Could you check a few things on this model? Use its own coordinates, in mm. Face numbers are marked on the shaded views. A direction names the side the tool comes from. Give positions to 0.01 mm unless a question says otherwise; leave off trailing zeros. One line per question, with ' | ' between items.
from build123d import *

# Parameters (mm, degrees)
BOSS_EXTRUDE1_DEPTH     = 6.2
BOSS_EXTRUDE3_DEPTH     = 6.2
CUT_EXTRUDE5_DEPTH      = 59.510170056
CUT_EXTRUDE5_DEPTH_BACK = 59.510170056
SKETCH9_W               = 8.426821026
SKETCH9_H               = 53.817918331
CUT_EXTRUDE6_DEPTH      = 56.427921054
CUT_EXTRUDE6_DEPTH_BACK = 56.427921054
SKETCH10_W              = 41.255234225
SKETCH10_H              = 19.128366746


with BuildPart() as part:
    # Sketch1 → Boss-Extrude1 (new body)
    with BuildSketch(Plane.XY):
        with BuildLine():
            Line((-28, 0), (0, 0))
            Line((0, 0), (0, 10))
            Line((0, 10), (-7.1, 10))
            ThreePointArc((-7.1, 10), (-14.171067812, 12.928932188), (-17.1, 20))
            Line((-17.1, 20), (-17.1, 51))
            Line((-17.1, 51), (-20.1, 51))
            Line((-20.1, 51), (-20.1, 6))
            Line((-20.1, 6), (-24, 6))
            Line((-24, 6), (-24, 50))
            Line((-24, 50), (-28, 50))
            Line((-28, 50), (-28, 0))
        make_face()
    extrude(amount=BOSS_EXTRUDE1_DEPTH)

    # Sketch7 → Boss-Extrude3 (add)
    with BuildSketch(Plane.XY.offset(6.2)):
        with BuildLine():
            Line((-16.7, 50.6), (-15.7, 50.5))
            ThreePointArc((-15.7, 50.5), (-15.462165524, 50.365875857), (-15.4, 50.1))
            ThreePointArc((-15.4, 50.1), (-15.462165524, 49.834124143), (-15.7, 49.7))
            Line((-15.7, 49.7), (-16.7, 49.6))
            ThreePointArc((-16.7, 49.6), (-16.971392676, 49.471392676), (-17.1, 49.2))
            Line((-17.1, 49.2), (-17.1, 48.75))
            ThreePointArc((-17.1, 48.75), (-16.971392676, 48.478607324), (-16.7, 48.35))
            Line((-16.7, 48.35), (-15.7, 48.25))
            ThreePointArc((-15.7, 48.25), (-15.462165524, 48.115875857), (-15.4, 47.85))
            ThreePointArc((-15.4, 47.85), (-15.462165524, 47.584124143), (-15.7, 47.45))
            Line((-15.7, 47.45), (-16.7, 47.35))
            ThreePointArc((-16.7, 47.35), (-16.971392676, 47.221392676), (-17.1, 46.95))
            Line((-17.1, 46.95), (-17.1, 46.5))
            ThreePointArc((-17.1, 46.5), (-16.971392676, 46.228607324), (-16.7, 46.1))
            Line((-16.7, 46.1), (-15.7, 46))
            ThreePointArc((-15.7, 46), (-15.462165524, 45.865875857), (-15.4, 45.6))
            ThreePointArc((-15.4, 45.6), (-15.462165524, 45.334124143), (-15.7, 45.2))
            Line((-15.7, 45.2), (-16.7, 45.1))
            ThreePointArc((-16.7, 45.1), (-16.971392676, 44.971392676), (-17.1, 44.7))
            Line((-17.1, 44.7), (-17.1, 44.25))
            ThreePointArc((-17.1, 44.25), (-16.971392676, 43.978607324), (-16.7, 43.85))
            Line((-16.7, 43.85), (-15.7, 43.75))
            ThreePointArc((-15.7, 43.75), (-15.462165524, 43.615875857), (-15.4, 43.35))
            ThreePointArc((-15.4, 43.35), (-15.462165524, 43.084124143), (-15.7, 42.95))
            Line((-15.7, 42.95), (-16.7, 42.85))
            ThreePointArc((-16.7, 42.85), (-16.971392676, 42.721392676), (-17.1, 42.45))
            Line((-17.1, 42.45), (-17.1, 42))
            ThreePointArc((-17.1, 42), (-16.971392676, 41.728607324), (-16.7, 41.6))
            Line((-16.7, 41.6), (-15.7, 41.5))
            ThreePointArc((-15.7, 41.5), (-15.462165524, 41.365875857), (-15.4, 41.1))
            ThreePointArc((-15.4, 41.1), (-15.462165524, 40.834124143), (-15.7, 40.7))
            Line((-15.7, 40.7), (-16.7, 40.6))
            ThreePointArc((-16.7, 40.6), (-16.971392676, 40.471392676), (-17.1, 40.2))
            Line((-17.1, 40.2), (-17.1, 39.75))
            ThreePointArc((-17.1, 39.75), (-16.971392676, 39.478607324), (-16.7, 39.35))
            Line((-16.7, 39.35), (-15.7, 39.25))
            ThreePointArc((-15.7, 39.25), (-15.462165524, 39.115875857), (-15.4, 38.85))
            ThreePointArc((-15.4, 38.85), (-15.462165524, 38.584124143), (-15.7, 38.45))
            Line((-15.7, 38.45), (-16.7, 38.35))
            ThreePointArc((-16.7, 38.35), (-16.971392676, 38.221392676), (-17.1, 37.95))
            Line((-17.1, 37.95), (-17.1, 37.5))
            ThreePointArc((-17.1, 37.5), (-16.971392676, 37.228607324), (-16.7, 37.1))
            Line((-16.7, 37.1), (-15.7, 37))
            ThreePointArc((-15.7, 37), (-15.462165524, 36.865875857), (-15.4, 36.6))
            ThreePointArc((-15.4, 36.6), (-15.462165524, 36.334124143), (-15.7, 36.2))
            Line((-15.7, 36.2), (-16.7, 36.1))
            ThreePointArc((-16.7, 36.1), (-16.971392676, 35.971392676), (-17.1, 35.7))
            Line((-17.1, 35.7), (-17.1, 35.25))
            ThreePointArc((-17.1, 35.25), (-16.971392676, 34.978607324), (-16.7, 34.85))
            Line((-16.7, 34.85), (-15.7, 34.75))
            ThreePointArc((-15.7, 34.75), (-15.462165524, 34.615875857), (-15.4, 34.35))
            ThreePointArc((-15.4, 34.35), (-15.462165524, 34.084124143), (-15.7, 33.95))
            Line((-15.7, 33.95), (-16.7, 33.85))
            ThreePointArc((-16.7, 33.85), (-16.971392676, 33.721392676), (-17.1, 33.45))
            Line((-17.1, 33.45), (-17.1, 33))
            ThreePointArc((-17.1, 33), (-16.971392676, 32.728607324), (-16.7, 32.6))
            Line((-16.7, 32.6), (-15.7, 32.5))
            ThreePointArc((-15.7, 32.5), (-15.462165524, 32.365875857), (-15.4, 32.1))
            ThreePointArc((-15.4, 32.1), (-15.462165524, 31.834124143), (-15.7, 31.7))
            Line((-15.7, 31.7), (-16.7, 31.6))
            ThreePointArc((-16.7, 31.6), (-16.971392676, 31.471392676), (-17.1, 31.2))
            Line((-17.1, 31.2), (-17.1, 30.75))
            ThreePointArc((-17.1, 30.75), (-16.971392676, 30.478607324), (-16.7, 30.35))
            Line((-16.7, 30.35), (-15.7, 30.25))
            ThreePointArc((-15.7, 30.25), (-15.462165524, 30.115875857), (-15.4, 29.85))
            ThreePointArc((-15.4, 29.85), (-15.462165524, 29.584124143), (-15.7, 29.45))
            Line((-15.7, 29.45), (-16.7, 29.35))
            ThreePointArc((-16.7, 29.35), (-16.971392676, 29.221392676), (-17.1, 28.95))
            Line((-17.1, 28.95), (-17.1, 28.5))
            ThreePointArc((-17.1, 28.5), (-16.971392676, 28.228607324), (-16.7, 28.1))
            Line((-16.7, 28.1), (-15.7, 28))
            ThreePointArc((-15.7, 28), (-15.462165524, 27.865875857), (-15.4, 27.6))
            ThreePointArc((-15.4, 27.6), (-15.462165524, 27.334124143), (-15.7, 27.2))
            Line((-15.7, 27.2), (-16.7, 27.1))
            ThreePointArc((-16.7, 27.1), (-16.971392676, 26.971392676), (-17.1, 26.7))
            Line((-17.1, 26.7), (-17.1, 26.25))
            ThreePointArc((-17.1, 26.25), (-16.971392676, 25.978607324), (-16.7, 25.85))
            Line((-16.7, 25.85), (-15.7, 25.75))
            ThreePointArc((-15.7, 25.75), (-15.462165524, 25.615875857), (-15.4, 25.35))
            ThreePointArc((-15.4, 25.35), (-15.462165524, 25.084124143), (-15.7, 24.95))
            Line((-15.7, 24.95), (-16.7, 24.85))
            ThreePointArc((-16.7, 24.85), (-16.971392676, 24.721392676), (-17.1, 24.45))
            Line((-17.1, 24.45), (-17.1, 24))
            ThreePointArc((-17.1, 24), (-16.971392676, 23.728607324), (-16.7, 23.6))
            Line((-16.7, 23.6), (-15.7, 23.5))
            ThreePointArc((-15.7, 23.5), (-15.462165524, 23.365875857), (-15.4, 23.1))
            ThreePointArc((-15.4, 23.1), (-15.462165524, 22.834124143), (-15.7, 22.7))
            Line((-15.7, 22.7), (-16.7, 22.6))
            ThreePointArc((-16.7, 22.6), (-16.971392676, 22.471392676), (-17.1, 22.2))
            Line((-17.1, 22.2), (-17.1, 21.75))
            ThreePointArc((-17.1, 21.75), (-16.971392676, 21.478607324), (-16.7, 21.35))
            Line((-16.7, 21.35), (-15.7, 21.25))
            ThreePointArc((-15.7, 21.25), (-15.462165524, 21.115875857), (-15.4, 20.85))
            ThreePointArc((-15.4, 20.85), (-15.462165524, 20.584124143), (-15.7, 20.45))
            Line((-15.7, 20.45), (-16.7, 20.35))
            ThreePointArc((-16.7, 20.35), (-16.971392676, 20.221392676), (-17.1, 19.95))
            Line((-17.1, 19.95), (-17.956542174, 50.55))
            Line((-17.956542174, 50.55), (-17.1, 51))
            ThreePointArc((-17.1, 51), (-16.971392676, 50.728607324), (-16.7, 50.6))
        make_face()
    extrude(amount=-BOSS_EXTRUDE3_DEPTH)

    # Sketch9 → Cut-Extrude5 (cut, two sides: drawn at the far end of the back side and taken through both)
    with BuildSketch(Plane.XY.offset(6.2).offset(-CUT_EXTRUDE5_DEPTH_BACK)):
        with Locations((-25.017603177, 24.82792225)):
            Rectangle(SKETCH9_W, SKETCH9_H)
    extrude(amount=CUT_EXTRUDE5_DEPTH + CUT_EXTRUDE5_DEPTH_BACK, mode=Mode.SUBTRACT)

    # Sketch10 → Cut-Extrude6 (cut, two sides: drawn at the far end of the back side and taken through both)
    with BuildSketch(Plane.XY.offset(6.2).offset(-CUT_EXTRUDE6_DEPTH_BACK)):
        with Locations((-9.089657701, 8.103525919)):
            Rectangle(SKETCH10_W, SKETCH10_H)
    extrude(amount=CUT_EXTRUDE6_DEPTH + CUT_EXTRUDE6_DEPTH_BACK, mode=Mode.SUBTRACT)


solid = part.part
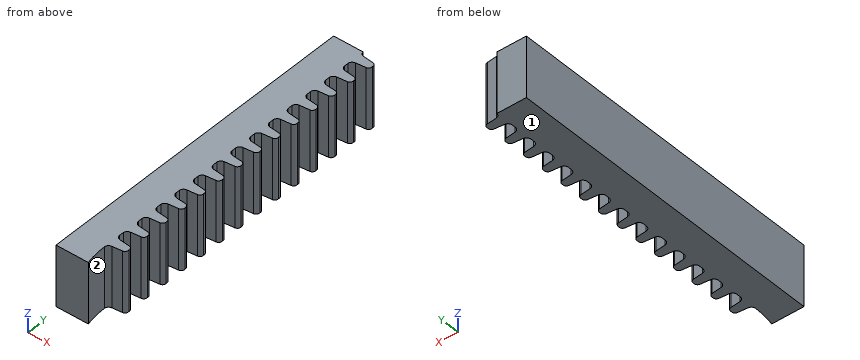
Q1. Will these pins go through, and if not, where does the flat tip stop? pin 1 (0.5 mm diameter, centred on y = 42, z = 3, fed in from +X); pin 2 (0.5 mm diameter, centred on y = 26.5, z = 3, fed in from +X); pin 3 (2 mm diameter, centred on x = -16.5, y = 28, fed in from -Z); pin 4 (1 mm diameter, centred on y = 31.5, z = 1, fed in from +X).
Answer below:
pin 1: stops at x = -16.99 | pin 2: stops at x = -17.09 | pin 3: stops at z = 0 | pin 4: stops at x = -15.4
Q2. If I drill on line 1 along X through (y, z) = (24, 2.5); line 2 along X through (y, z) = (27, 3.5), over which ranges is the centre line in solid material (lowest first)?
Answer below:
line 1: x = -20.1 to -17.1 | line 2: x = -20.1 to -16.94
Q3. Imagine slicing it at A-A on x = -16. Count the separate pieces of the cut face and the enclosed holes in it, and give its area (3 significant figures).
Answer below:
separate pieces: 14 | enclosed holes: 0 | area: 74.6 mm^2
Q4. On a 3-axis mill with a long thin cutter (end or side, diameter ignored), from which of +Z, -Z, +X, -X, +Y, -Y can I reach the whole of each face in a straight line? I mean the marked faces 1 and 2. Say none if no direction works.
Answer below:
face 1: -Z, +X, -X, +Y, -Y | face 2: +Z, -Z, +X
